Could you check a few things on this model? Use its own coordinates, in mm. A direction names the side the tool comes from. Coordinates: 2 decimals unless noted, no trailing zeros. Order: outer loops, then holes, each group sorted by start corner. A loop starts at its lowest first (then second) coordinate and runs counter-clockwise, first axis right, second up. Notation, with made-up numbers: (22, 73) - (75, 73) arc R14 cw to (75, 79) - close; hole circle Ø3 at (74.25, -28.5). An arc over 180 degrees is marked (long way). Answer as CSV lines item,"result". Start each with the question number.
1. Thinking about a two-plate mould opening in Y: for faces 1 (the face through (20, 4, 0)), 2 (the face through (20, 40, 1)), 3 (the face through (8.452, -8.581, 1.479)), which applies, released by +Y, released by -Y, zero draft, split by the parting line, or undercut?
2. I want a section at B-B, the plane y = -10. List the corners of the cut face in (x, z) for me, and give its area (3 significant figures).
3. I want a section at A-A, the plane z = 0.9. Count the separate pieces of the cut face and the enclosed holes in it, and give its area (3 significant figures).
4. I need wall thicknesses on probe 1 along Y at (x, z) = (20, 1.2); probe 2 along X at (y, z) = (-8.5, 0.2); probe 3 along Y at (x, z) = (21, 2.75). Which ranges of each line are inside material? Lowest first, please.
5. For pin 1 (2.5 mm diameter, centred on x = 20, y = -10, fed in from +Z); pin 2 (1.5 mm diameter, centred on y = 14, z = 2, fed in from -X), each with a flat end and sliding along its axis, tell me the tip position at first contact or that it passes through.
6. I want a section at C-C, the plane y = 10. List the corners of the cut face in (x, z) for me.
7. I want a section at D-D, the plane y = 24.5. List the corners of the cut face in (x, z) for me.
8. For faces 4 (the face through (30, 20, 1)), 5 (the face through (10, 20, 1)), 6 (the face through (20.969, 28.137, 1.479)), which set-ups out of +Z, -Z, +X, -X, +Y, -Y let a thin tool reach every point of the face, with its end or its side?
from build123d import *

# Parameters (mm, degrees)
SKETCH_1_R      = 2.1
EXTRUDE_1_DEPTH = 3
FILLET_1_R      = 5
FILLET_2_R      = 5


with BuildPart() as part:
    # 草图1 → 凸台-拉伸1 (new body)
    with BuildSketch(Plane.XY):
        Polygon((10, 0), (10, 40), (30, 40), (30, 0), (40, 0), (40, -20), (0, -20), (0, 0), align=None)
        with Locations((20, -10)):
            Circle(SKETCH_1_R, mode=Mode.SUBTRACT)
        with Locations((10, -10)):
            Circle(SKETCH_1_R, mode=Mode.SUBTRACT)
        with Locations((30, -10)):
            Circle(SKETCH_1_R, mode=Mode.SUBTRACT)
        with Locations((20, 10)):
            Circle(SKETCH_1_R, mode=Mode.SUBTRACT)
        with Locations((20, 30)):
            Circle(SKETCH_1_R, mode=Mode.SUBTRACT)
    extrude(amount=EXTRUDE_1_DEPTH)

    # 圆角1
    fillet_1_edges = [part.edges().sort_by_distance(p)[0] for p in [
        (10, 40, 1.5),
        (30, 40, 1.5),
        (40, -20, 1.5),
        (40, 0, 1.5),
        (30, 0, 1.5),
        (10, 0, 1.5),
        (0, 0, 1.5),
    ]]
    fillet(fillet_1_edges, radius=FILLET_1_R - 0.0001)  # a hair under: the kernel refuses the full size

    # 圆角2
    fillet_2_edges = [part.edges().sort_by_distance(p)[0] for p in [
        (0, -20, 1.5),
    ]]
    fillet(fillet_2_edges, radius=FILLET_2_R)


solid = part.part
Solved:
1,face 1,"zero draft"
1,face 2,"released by +Y"
1,face 3,"undercut"
2,outline,"(0, 0) - (7.9, 0) - (7.9, 3) - (0, 3) - close; (12.1, 0) - (17.9, 0) - (17.9, 3) - (12.1, 3) - close; (22.1, 0) - (27.9, 0) - (27.9, 3) - (22.1, 3) - close; (32.1, 0) - (40, 0) - (40, 3) - (32.1, 3) - close"
2,area,"82.2 mm2"
3,separate pieces,"1"
3,enclosed holes,"5"
3,area,"1,510 mm2"
4,probe 1,"y = -20 to -12.1, -7.9 to 7.9, 12.1 to 27.9, 32.1 to 40"
4,probe 2,"x = 0 to 8.53, 11.47 to 18.53, 21.47 to 28.53, 31.47 to 40"
4,probe 3,"y = -20 to -11.85, -8.15 to 8.15, 11.85 to 28.15, 31.85 to 40"
5,pin 1,"passes through"
5,pin 2,"stops at x = 10"
6,outline,"(10, 0) - (17.9, 0) - (17.9, 3) - (10, 3) - close; (22.1, 0) - (30, 0) - (30, 3) - (22.1, 3) - close"
7,outline,"(10, 0) - (30, 0) - (30, 3) - (10, 3) - close"
8,face 4,"+Z, -Z, +X, +Y"
8,face 5,"+Z, -Z, -X, +Y"
8,face 6,"+Z, -Z"
